Geometry check sheet. Reference: the model listing, model coordinates, mm. A direction names the side the tool comes from. Give positions to 0.01 mm unless a question says otherwise; leave off trailing zeros. Write each loop counter-clockwise with the first axis right and the second up, starting at its lowest first coordinate (ties: lowest second). Pieces come first, ordered by that corner, then holes. Notation, with made-up numbers: (18.25, -18.75) - (53.25, -18.75) arc R32 cw to (53.25, 15.25) - close; hole circle Ø2 at (16.25, -38.5). An arc over 180 degrees is marked (long way). Use a Markdown table: item, result.
```python
from build123d import *

# Parameters (mm, degrees)
SKETCH1_W                   = 101.6
SKETCH1_H                   = 12.7
BOSS_EXTRUDE1_DEPTH         = 12.7
F_32_0_116_DIAMETER_HOLE1_D = 2.9464
SKETCH5_W                   = 101.6
SKETCH5_H                   = 7.112
BOSS_EXTRUDE2_DEPTH         = 2.54


with BuildPart() as part:
    # Sketch1 → Boss-Extrude1 (new body)
    with BuildSketch(Plane(origin=(0, 0, 0), x_dir=(1, 0, 0), z_dir=(0, 1, 0))):
        with Locations((50.8, 6.35)):
            Rectangle(SKETCH1_W, SKETCH1_H)
    extrude(amount=BOSS_EXTRUDE1_DEPTH)

    # #32 (0.116) Diameter Hole1 (through all)
    with Locations(Plane(origin=(0, 12.7, 0), x_dir=(1, 0, 0), z_dir=(0, 1, 0))):
        with Locations((6.35, 6.35), (95.25, 6.35)):
            Hole(F_32_0_116_DIAMETER_HOLE1_D / 2)

    # Sketch5 → Boss-Extrude2 (add)
    with BuildSketch(Plane.XY):
        with Locations((50.8, 3.556)):
            Rectangle(SKETCH5_W, SKETCH5_H)
    extrude(amount=BOSS_EXTRUDE2_DEPTH)


solid = part.part
```
1) Material ranges on L1, parallel to X at y = 7.75, z = -6.35; L2, parallel to Z at x = 6.35, y = 4.75; L3, parallel to X at y = 6, z = -7.5, recorded low to high. Write a range as from..to.
Working result:
| item | result |
|---|---|
| L1 | x = 0..4.88, 7.82..93.78, 96.72..101.6 |
| L2 | z = -12.7..-7.82, -4.88..2.54 |
| L3 | x = 0..5.43, 7.27..94.33, 96.17..101.6 |
2) Set-up check for faces 5 (the flat face through (50, 10, 0)), 6 (the flat face through (50, 0, -5)): record each of +Z, -Z, +X, -X, +Y, -Y from which the full face is reachable in a straight line by a thin tool's end or side.
Working result:
| item | result |
|---|---|
| face 5 | +Z, +X, -X, +Y |
| face 6 | +Z, -Z, +X, -X, -Y |
3) Mould release check, pull along Z, two halves, no side actions. Record for faces 1 (the cylindrical face through (7.436, 6.261, -7.346)), 2 (the cylindrical face through (93.845, 6.261, -6.793)), 3 (the flat face through (0, 6, -5)), 4 (the flat face through (50, 4, 2.54)): pulls with the +Z half, pulls with the -Z half, needs draft (parallel to the pull), parting line crosses it, or undercut.
Working result:
| item | result |
|---|---|
| face 1 | undercut |
| face 2 | undercut |
| face 3 | needs draft |
| face 4 | pulls with the +Z half |
4) Section check A-A on x = 95.25. Record the boundary of the cut face in (y, z), then the cut area to 3 significant figures.
Working result:
| item | result |
|---|---|
| outline | (0, -12.7) - (12.7, -12.7) - (12.7, -7.82) - (0, -7.82) - close; (0, -4.88) - (12.7, -4.88) - (12.7, 0) - (7.11, 0) - (7.11, 2.54) - (0, 2.54) - close |
| area | 142 mm² |
5) Depth check by flat-ended pin: P1, Ø1.3, axis at x = 55.5, z = 2, coming from the +Y side; P2, Ø2.5, axis at x = 6.35, z = -6.35, coming from the -Y side. Enter the tip coordinate at first touch or a pass-through.
Working result:
| item | result |
|---|---|
| P1 | stops at y = 7.11 |
| P2 | passes through |
6) Section check B-B on z = -6.35. Record the boundary of the cut face in (x, y), then the cut area to 3 significant figures.
Working result:
| item | result |
|---|---|
| outline | (0, 0) - (4.88, 0) - (4.88, 12.7) - (0, 12.7) - close; (7.82, 0) - (93.78, 0) - (93.78, 12.7) - (7.82, 12.7) - close; (96.72, 0) - (101.6, 0) - (101.6, 12.7) - (96.72, 12.7) - close |
| area | 1,220 mm² |
7) Section check C-C on x = 31.5. Record the boundary of the cut face in (y, z), then the cut area to 3 significant figures.
Working result:
| item | result |
|---|---|
| outline | (0, -12.7) - (12.7, -12.7) - (12.7, 0) - (7.11, 0) - (7.11, 2.54) - (0, 2.54) - close |
| area | 179 mm² |
